Geometry check sheet. Reference: the model listing, model coordinates, mm. Give positions to 0.01 mm unless a question says otherwise; leave off trailing zeros. Order: outer loops, then holes, each group sorted by start corner. A loop starts at its lowest first (then second) coordinate and runs counter-clockwise, first axis right, second up.
```python
from build123d import *

# Parameters (mm, degrees)
SKETCH1_R      = 4.8
TUBE_DEPTH     = 20
SKETCH3_R      = 0.6
SKETCH6_R      = 0.6
SKETCH9_R      = 0.45
SKETCH10_R     = 0.45
SKETCH11_W     = 12.950895794
SKETCH11_H     = 9.583916724
WIRE_CUT_DEPTH = 5


with BuildPart() as part:
    # Sketch1 → Tube (new body)
    with BuildSketch(Plane(origin=(0, 0, 0), x_dir=(0, 0, -1), z_dir=(1, 0, 0))):
        Circle(SKETCH1_R)
    extrude(amount=TUBE_DEPTH)

    # Sweep1: sweep along a path in Sketch2
    with BuildLine(Plane(origin=(0, 0, 0), x_dir=(1, 0, 0), z_dir=(0, 1, 0))) as sweep1_path:
        Line((20, 0.437533256), (39.938874032, 2))
    # Sketch3 → Sweep1 (sweep)
    with BuildSketch(Plane(origin=(20, 0, 0), x_dir=(0, 0, -1), z_dir=(1, 0, 0))):
        with Locations((0.437533256, 0)):
            Circle(SKETCH3_R)
    sweep(path=sweep1_path.line)

    # Sweep2: sweep along a path in Sketch5
    with BuildLine(Plane(origin=(0, 0, 0), x_dir=(1, 0, 0), z_dir=(0, 1, 0))) as sweep2_path:
        Line((20, -1.392543459), (39.452849812, -2))
    # Sketch6 → Sweep2 (sweep)
    with BuildSketch(Plane(origin=(20, 0, 0), x_dir=(0, 0, -1), z_dir=(1, 0, 0))):
        with Locations((-1.392543459, 0)):
            Circle(SKETCH6_R)
    sweep(path=sweep2_path.line)

    # ca: sweep along a path in Sketch7
    with BuildLine(Plane(origin=(0, 0, 0), x_dir=(1, 0, 0), z_dir=(0, 1, 0))) as ca_path:
        Line((39.938874032, 2), (52.603130391, 2.998856902))
    # Sketch9 → ca (sweep)
    with BuildSketch(Plane(origin=(39.938874032, 0, 0), x_dir=(0, 0, -1), z_dir=(1, 0, 0))):
        with Locations((2, 0)):
            Circle(SKETCH9_R)
    sweep(path=ca_path.line)

    # an: sweep along a path in Sketch8
    with BuildLine(Plane(origin=(0, 0, 0), x_dir=(1, 0, 0), z_dir=(0, 1, 0))) as an_path:
        Line((39.452849812, -2), (53.102297824, -2.764258006))
    # Sketch10 → an (sweep)
    with BuildSketch(Plane(origin=(39.452849812, 0, 0), x_dir=(0, 0, -1), z_dir=(1, 0, 0))):
        with Locations((-2, 0)):
            Circle(SKETCH10_R)
    sweep(path=an_path.line)

    # Sketch11 → wire cut (cut, symmetric)
    with BuildSketch(Plane(origin=(0, 0, 0), x_dir=(1, 0, 0), z_dir=(0, 1, 0))):
        with Locations((48.578158556, -0.027699181)):
            Rectangle(SKETCH11_W, SKETCH11_H)
    extrude(amount=WIRE_CUT_DEPTH, both=True, mode=Mode.SUBTRACT)


solid = part.part
```
Q1. Release check for a two-part mould opening along X. For faces 1 (the face through (9.86, 4.05, -2.58)), 2 (the face through (0, 0, 0)), 3 (the face through (42.103, 0, -2)) record: pulls with the +X half, pulls with the -X half, needs draft (parallel to the pull), parting line crosses it, or undercut.
Q2. Thickness scan on L1, parallel to X at y = 1, z = -3.25; L2, parallel to Y at x = 13.5, z = 3.75; L3, parallel to Z at x = 2, y = 1. Record the ranges inside material, lowest first.
Q3. Cross-section at B-B, the plane y = -2.75. Record the boundary of the cut face in (x, z).
Q4. Gauge pin test, flat ends, axial feed: P1, Ø5, axis at x = 23.5, y = 2, coming from the +Z side; P2, Ø5, axis at x = 30.5, z = -3.5, coming from the -Y side; P3, Ø3, axis at x = 19.5, z = -3, coming from the -Y side. Record the tip position at first contact, or that the pin passes through.
Q5. Cross-section at A-A, the plane x = 5.5. Record the boundary of the cut face in (y, z), and give its area (3 significant figures).
Answers follow:
1. face 1: needs draft
1. face 2: pulls with the -X half
1. face 3: pulls with the +X half
2. L1: x = 0 to 20
2. L2: y = -3 to 3
2. L3: z = -4.69 to 4.69
3. outline: (0, -3.93) - (20, -3.93) - (20, 3.93) - (0, 3.93) - close
4. P1: stops at z = 2.15
4. P2: stops at y = -0.6
4. P3: stops at y = -4.56
5. outline: circle Ø9.6 at (0, 0)
5. area: 72.4 mm2
